```python
from build123d import *

# Parameters (mm, degrees)
F1_DEPTH = 146.001203


with BuildPart() as f1:
    # F0 (on Right) → F1 (new body)
    with BuildSketch(Plane.YZ):
        with BuildLine():
            Line((38.369116, 72.40589), (-18.330798, 72.40589))
            Line((-18.330798, 72.40589), (-18.330798, -30.96252))
            ThreePointArc((-18.330798, -30.96252), (-11.754066, -46.840154), (4.123567, -53.416885))
            Line((4.123567, -53.416885), (53.274147, -53.416885))
            Line((53.274147, -53.416885), (53.274147, 57.500858))
            ThreePointArc((53.274147, 57.500858), (48.908565, 68.040307), (38.369116, 72.40589))
        make_face()
    extrude(amount=F1_DEPTH)


solid = f1.part
```
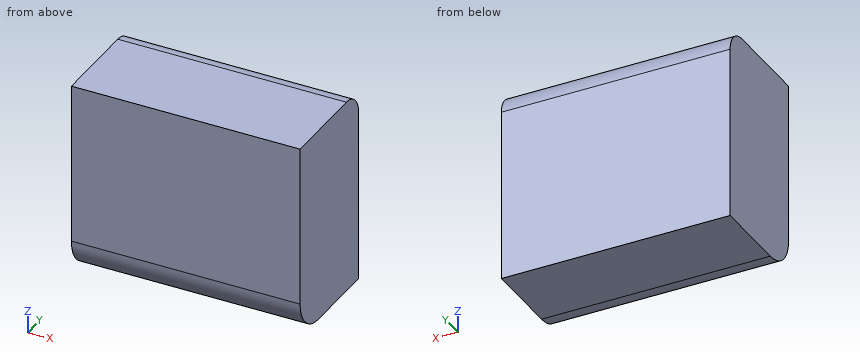
The model under review builds one solid part; all positions refer to its coordinate system, in mm. Round coordinates to 2 decimals unless told otherwise and drop trailing zeros. Write each loop counter-clockwise with the first axis right and the second up, starting at its lowest first coordinate (ties: lowest second). Pieces come first, ordered by that corner, then holes.
(1) We need section A-A on x = 78. Give the boundary of the cut face in (y, z).
(2) We need section C-C on y = 48. Give the boundary of the cut face in (x, z).
(3) Wall thickness on L1, parallel to Z at x = 33, y = 38.5; L2, parallel to Z at x = 121.5, y = 46; L3, parallel to Y at x = 12.5, z = -45: over which ranges is each line inside the solid? List them lowest first.
(4) We need section B-B on y = -5. Give the boundary of the cut face in (x, z), and give its area (3 significant figures).
Findings below:
1. outline: (-18.33, -30.96) arc R22.45 ccw to (4.12, -53.42) - (53.27, -53.42) - (53.27, 57.5) arc R14.91 ccw to (38.37, 72.41) - (-18.33, 72.41) - close
2. outline: (0, -53.42) - (146, -53.42) - (146, 68.88) - (0, 68.88) - close
3. L1: z = -53.42 to 72.41
3. L2: z = -53.42 to 70.3
3. L3: y = -13.4 to 53.27
4. outline: (0, -51.48) - (146, -51.48) - (146, 72.41) - (0, 72.41) - close
4. area: 18,100 mm2
